Here's the drawing with two shaded views (mm, measured from the low corner). I have some questions. Give positions to 0.01 mm unless a question says otherwise; leave off trailing zeros. Loops run counter-clockwise (first coordinate to the right, second up) from the corner with the lowest first, then second, coordinate; pieces in that order, holes last. Notation, with made-up numbers: (19, 61) -> (43, 61) arc R21 ccw to (43, 75) -> close; hole circle Ø5 at (67, 82.25). An arc over 180 degrees is marked (long way). Answer in a Markdown table with one row per item. Add a question column.
Item 1: If we section it at C-C (x = 65.5): Write out the boundary of the cut face in (y, z).
Item 2: If we section it at B-B (z = 263): Write out the boundary of the cut face in (x, y), then the cut area to 4 significant figures.
Item 3: For P1, Ø2.5, axis at x = 38, y = 46.5, coming from the +Z side; P2, Ø3, axis at x = 10, z = 40.5, coming from the +Y side; P3, Ø5, axis at x = 13.5, y = 29, coming from the +Z side; P4, Ø3.5, axis at x = 27.5, y = 46.5, coming from the -Z side, each with a flat end and sliding along its axis, tell me the tip position at first contact or that it passes through.
Item 4: If I drill on line 1 (Y direction, x = 36, z = 133.5); line 2 (Z direction, x = 56, y = 42); line 3 (Z direction, x = 8.5, y = 36) (1 decimal), over which ranges is the centre line in solid material (lowest first)?
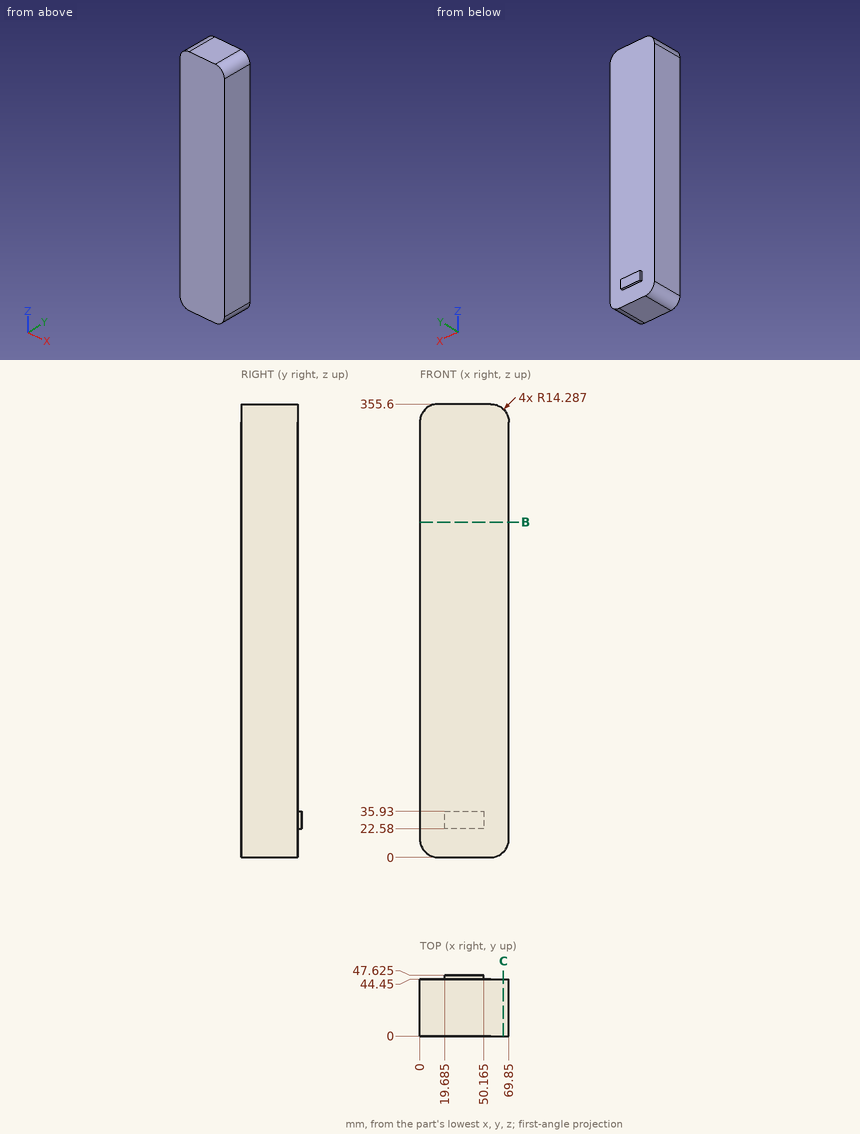
Recorded:
| question | item | result |
|---|---|---|
| 1 | outline | (0, 4.02) -> (44.45, 4.02) -> (44.45, 351.58) -> (0, 351.58) -> close |
| 2 | outline | (0, 0) -> (69.85, 0) -> (69.85, 44.45) -> (0, 44.45) -> close |
| 2 | area | 3,105 mm^2 |
| 3 | P1 | stops at z = 35.93 |
| 3 | P2 | stops at y = 44.45 |
| 3 | P3 | stops at z = 355.6 |
| 3 | P4 | stops at z = 22.58 |
| 4 | line 1 | y = 0 to 44.45 |
| 4 | line 2 | z = 0.01 to 355.59 |
| 4 | line 3 | z = 1.2 to 354.4 |
